from build123d import *

# Parameters (mm, degrees)
SKETCH1_R              = 4
BOSS_EXTRUDE1_DEPTH    = 27.5
SKETCH2_W              = 61.091432286
SKETCH2_H              = 28.689736928
CUT_EXTRUDE1_DEPTH     = 25
SKETCH3_R              = 4
BOSS_EXTRUDE2_DEPTH    = 35
SKETCH4_W              = 71.474314091
SKETCH4_H              = 50
CUT_EXTRUDE2_DEPTH     = 79.778169565
SHELL1_START           = -25.5
SHELL1_DEPTH           = 51
SHELL1_START_2         = -33
SHELL1_2_OUTLINE_R     = 2
SHELL1_2_DEPTH         = 66
SKETCH5_W              = 18
SKETCH5_H              = 15
CUT_EXTRUDE3_DEPTH     = 92.752384165
FILLET1_R              = 2
LPATTERN1_COUNT        = 3
LPATTERN1_PITCH        = 30
FILLET1_OF_LPATTERN1_R = 2


# Read off the part's stored shape, not the designer's step: Shell1
with BuildPart() as part:
    # Sketch1 → Boss-Extrude1 (new, symmetric)
    with BuildSketch(Plane.XY):
        with BuildLine():
            Line((-53.5, 12.5), (53.5, 12.5))
            ThreePointArc((53.5, 12.5), (66, 0), (53.5, -12.5))
            Line((53.5, -12.5), (-53.5, -12.5))
            ThreePointArc((-53.5, -12.5), (-66, 0), (-53.5, 12.5))
        make_face()
        with Locations((53.5, 0)):
            Circle(SKETCH1_R, mode=Mode.SUBTRACT)
    extrude(amount=BOSS_EXTRUDE1_DEPTH, both=True)

    # Sketch2 → Cut-Extrude1 (cut, symmetric)
    with BuildSketch(Plane.XY):
        with Locations((53.5, 0)):
            Rectangle(SKETCH2_W, SKETCH2_H)
    extrude(amount=CUT_EXTRUDE1_DEPTH, both=True, mode=Mode.SUBTRACT)

    # Sketch3 → Boss-Extrude2 (add, symmetric)
    with BuildSketch(Plane.XY):
        with Locations((-53.5, 0)):
            Circle(SKETCH3_R)
    extrude(amount=BOSS_EXTRUDE2_DEPTH, both=True)

    # Sketch4 → Cut-Extrude2 (cut, through all)
    with BuildSketch(Plane(origin=(0, 12.5, 0), x_dir=(1, 0, 0), z_dir=(0, 1, 0))):
        with Locations((-12.782873189, 0)):
            Rectangle(SKETCH4_W, SKETCH4_H)
    extrude(amount=-CUT_EXTRUDE2_DEPTH, mode=Mode.SUBTRACT)

    # Shell1 outline → Shell1 (cut)
    with BuildSketch(Plane.XY.offset(SHELL1_START)):
        with BuildLine():
            Line((-48.520030234, -10.5), (-48.520030234, 10.5))
            Line((-48.520030234, 10.5), (-53.5, 10.5))
            ThreePointArc((-53.5, 10.5), (-64, 0), (-53.5, -10.5))
            Line((-53.5, -10.5), (-48.520030234, -10.5))
        make_face()
    extrude(amount=SHELL1_DEPTH, mode=Mode.SUBTRACT)

    # Shell1 2 outline → Shell1 2 (cut)
    with BuildSketch(Plane.XY.offset(SHELL1_START_2)):
        with Locations((-53.5, 0)):
            Circle(SHELL1_2_OUTLINE_R)
    extrude(amount=SHELL1_2_DEPTH, mode=Mode.SUBTRACT)

    # Sketch5 → Cut-Extrude3 (cut, through all)
    with BuildSketch(Plane.XY.offset(27.5)):
        with Locations((-31.5, 0)):
            Rectangle(SKETCH5_W, SKETCH5_H)
    cut_extrude3 = extrude(amount=-CUT_EXTRUDE3_DEPTH, mode=Mode.SUBTRACT)

    # Fillet1
    fillet1_edges = [part.edges().sort_by_distance(p)[0] for p in [
        (-40.5, -7.5, -26.25),
        (-40.5, -7.5, 26.25),
        (-40.5, 7.5, -26.25),
        (-40.5, 7.5, 26.25),
        (-22.5, 7.5, -26.25),
        (-22.5, 7.5, 26.25),
        (-22.5, -7.5, -26.25),
        (-22.5, -7.5, 26.25),
    ]]
    fillet(fillet1_edges, radius=FILLET1_R)

    # LPattern1: Cut-Extrude3 ×3
    with Locations(*[(i * LPATTERN1_PITCH, 0, 0) for i in range(1, LPATTERN1_COUNT)]):
        add(cut_extrude3, mode=Mode.SUBTRACT)

    # Fillet1 of LPattern1
    fillet1_of_lpattern1_edges = [part.edges().sort_by_distance(p)[0] for p in [
        (-10.5, -7.5, -26.25),
        (-10.5, -7.5, 26.25),
        (-10.5, 7.5, -26.25),
        (-10.5, 7.5, 26.25),
        (7.5, 7.5, -26.25),
        (7.5, 7.5, 26.25),
        (7.5, -7.5, -26.25),
        (7.5, -7.5, 26.25),
        (19.5, -7.5, -26.25),
        (19.5, -7.5, 26.25),
        (19.5, 7.5, -26.25),
        (19.5, 7.5, 26.25),
        (37.5, 7.5, -26.25),
        (37.5, 7.5, 26.25),
        (37.5, -7.5, -26.25),
        (37.5, -7.5, 26.25),
    ]]
    fillet(fillet1_of_lpattern1_edges, radius=FILLET1_OF_LPATTERN1_R)


solid = part.part
Verification items for the finished model (mm, model axes). A direction names the side the tool comes from. Coordinates: 2 decimals unless noted, no trailing zeros. Loops run counter-clockwise (first coordinate to the right, second up) from the corner with the lowest first, then second, coordinate; pieces in that order, holes last. Notation, with made-up numbers: M 14.25,85 L 32.25,85 A17 ccw 32.25,115 Z; hole C 76,75 d3. An arc over 180 degrees is marked long. One line per item, written item: value.
1. Set-up check for faces 3 (the flat face through (-54, 0, 35)), 4 (the cylindrical face through (-55.498, 0.088, 29.197)), 5 (the flat face through (28, -7.5, -26)), 6 (the flat face through (8, 0, 25)): record each of +Z, -Z, +X, -X, +Y, -Y from which the full face is reachable in a straight line by a thin tool's end or side.
Answers follow:
face 3: +Z, +X, -X, +Y, -Y
face 4: none
face 5: +Z, -Z
face 6: +X, +Y, -Y
2. Section check B-B on z = 4. Record the cut outline in (x, y), plus the area to 3 significant figures.
Answers follow:
outline: M -53.5,-12.5 L -48.52,-12.5 L -48.52,-10.5 L -53.5,-10.5 A10.5 cw -53.5,10.5 L -48.52,10.5 L -48.52,12.5 L -53.5,12.5 A12.5 ccw Z
area: 92.2 mm^2
3. Gauge pin test, flat ends, axial feed: P1, Ø1.5, axis at x = -48.5, y = -8, coming from the -Z side; P2, Ø5, axis at y = -9, z = 26.5, coming from the +X side; P3, Ø1.5, axis at x = 15, y = 2, coming from the +Z side. Record the tip position at first contact, or that the pin passes through.
Answers follow:
P1: z = -27.5
P2: x = 64.18
P3: z = 27.5
4. Section check C-C on y = 0. Give the number of separate pieces and of enclosed holes in the cut face, plus the area to 3 significant figures.
Answers follow:
separate pieces: 9
enclosed holes: 0
area: 495 mm^2
5. Material ranges on line 1 along X through (y, z) = (0, -26.55); line 2 along Z through (x, y) = (-9, -10); line 3 along Z through (x, y) = (-49, 8), recorded low to high. Write a range as from..to.
Answers follow:
line 1: -66..-55.5, -51.5..-40.5, -22.5..-10.5, 7.5..19.5, 37.5..49.5, 57.5..66
line 2: -27.5..-25, 25..27.5
line 3: -27.5..-25.5, 25.5..27.5
6. Section check A-A on x = 2.5. Record the cut outline in (y, z), plus the area to 3 significant figures.
Answers follow:
outline: M -12.5,-27.5 L -7.5,-27.5 L -7.5,-25 L -12.5,-25 Z; M -12.5,25 L -7.5,25 L -7.5,27.5 L -12.5,27.5 Z; M 7.5,-27.5 L 12.5,-27.5 L 12.5,-25 L 7.5,-25 Z; M 7.5,25 L 12.5,25 L 12.5,27.5 L 7.5,27.5 Z
area: 50.0 mm^2
7. Mould release check, pull along X, two halves, no side actions. Record for faces 1 (the flat face through (8, 0, -25)), 2 (the flat face through (-56, 0, -25.5)): pulls with the +X half, pulls with the -X half, needs draft (parallel to the pull), parting line crosses it, or undercut.
Answers follow:
face 1: needs draft
face 2: undercut
